Geometry check sheet. Reference: the model listing, model coordinates, mm. Face numbers are marked on the shaded views. A direction names the side the tool comes from. Coordinates: 2 decimals unless noted, no trailing zeros. Order: outer loops, then holes, each group sorted by start corner. A loop starts at its lowest first (then second) coordinate and runs counter-clockwise, first axis right, second up. Notation, with made-up numbers: (19, 74) - (64, 74) arc R24 cw to (64, 97) - close; hole circle Ø9 at (15, -25.75). An arc over 180 degrees is marked (long way). Put each result on its own line as item: value.
from build123d import *

# Parameters (mm, degrees)
SKETCH4_R           = 37.5
BOSS_EXTRUDE2_DEPTH = 5
SKETCH5_R           = 8.5
CUT_EXTRUDE1_DEPTH  = 54.268189382
BOSS_EXTRUDE3_DEPTH = 4.7
SKETCH1_R           = 37.5
SKETCH1_R_2         = 26.5
CUT_EXTRUDE2_DEPTH  = 57.626164447


with BuildPart() as part:
    # Sketch4 → Boss-Extrude2 (new body)
    with BuildSketch(Plane.XY):
        Circle(SKETCH4_R)
    extrude(amount=BOSS_EXTRUDE2_DEPTH)

    # Sketch5 → Cut-Extrude1 (cut, through all)
    with BuildSketch(Plane.XY.offset(5)):
        Circle(SKETCH5_R)
    extrude(amount=-CUT_EXTRUDE1_DEPTH, mode=Mode.SUBTRACT)

    # Sketch6 → Boss-Extrude3 (add, symmetric)
    with BuildSketch(Plane(origin=(0, 0, 0), x_dir=(1, 0, 0), z_dir=(0, 1, 0))):
        Polygon((26.5, 0), (20.712132034, 0), (23.65, 2.937867966), (23.65, 14.562132034), (21.65, 16.562132034), (21.65, 19.85), (26.5, 19.85), align=None)
    boss_extrude3 = extrude(amount=BOSS_EXTRUDE3_DEPTH, both=True)

    # Mirror1: Boss-Extrude3 across plane
    add(boss_extrude3.mirror(Plane(origin=(0, 0, 0), x_dir=(0, 0, 1), z_dir=(1, 0, 0))))

    # Sketch1 → Cut-Extrude2 (cut, through all)
    with BuildSketch(Plane.XY):
        Circle(SKETCH1_R)
        Circle(SKETCH1_R_2, mode=Mode.SUBTRACT)
    extrude(amount=-CUT_EXTRUDE2_DEPTH, mode=Mode.SUBTRACT)


solid = part.part
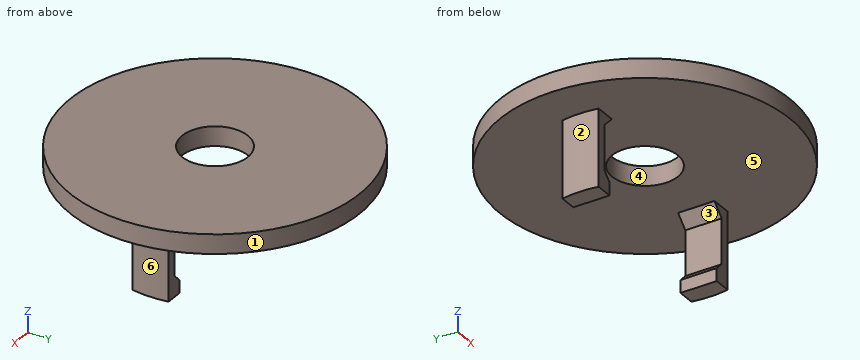
Q1. Thickness scan on L1, parallel to Y at x = 0, z = 3.85; L2, parallel to Z at x = 32, y = 1; L3, parallel to X at y = -1, z = -16.5. Record the ranges inside material, lowest first. Write a range as [from, to].
Answer block:
L1: y = [-37.5, -8.5], [8.5, 37.5]
L2: z = [0, 5]
L3: x = [-26.48, -21.71], [21.71, 26.48]
Q2. Section check B-B on z = -9.75. Record the boundary of the cut face in (x, y).
Answer block:
outline: (-26.08, -4.7) - (-23.65, -4.7) - (-23.65, 4.7) - (-26.08, 4.7) arc R26.5 ccw to start; (23.65, -4.7) - (26.08, -4.7) arc R26.5 ccw to (26.08, 4.7) - (23.65, 4.7) - close
Q3. Draft check along Y on the marked faces 4, 5 and 6. Enter one of: pulls with the +Y half, pulls with the -Y half, needs draft (parallel to the pull), parting line crosses it, or undercut.
Answer block:
face 4: undercut
face 5: needs draft
face 6: parting line crosses it
Q4. Section check A-A on x = 0. Record the boundary of the cut face in (y, z), then the cut area to 3 significant figures.
Answer block:
outline: (-37.5, 0) - (-8.5, 0) - (-8.5, 5) - (-37.5, 5) - close; (8.5, 0) - (37.5, 0) - (37.5, 5) - (8.5, 5) - close
area: 290 mm^2
Q5. Depth check by flat-ended pin: pin 1 Ø2.5 at (x, z) = (22.5, -7.5) entering from +Y; pin 2 Ø1.6 at (x, z) = (-24.5, -9.5) entering from -Y; pin 3 Ø12 at (x, y) = (-21.5, -27) entering from -Z; pin 4 Ø5 at (y, z) = (-19.5, -4.5) entering from -X. Enter the tip coordinate at first touch or a pass-through.
Answer block:
pin 1: stops at y = 4.7
pin 2: stops at y = -4.7
pin 3: stops at z = 0
pin 4: passes through
Q6. Section check C-C on y = 0. Record the boundary of the cut face in (x, z), then the cut area to 3 significant figures.
Answer block:
outline: (-37.5, 0) - (-26.5, 0) - (-26.5, -19.85) - (-21.65, -19.85) - (-21.65, -16.56) - (-23.65, -14.56) - (-23.65, -2.94) - (-20.71, 0) - (-8.5, 0) - (-8.5, 5) - (-37.5, 5) - close; (8.5, 0) - (20.71, 0) - (23.65, -2.94) - (23.65, -14.56) - (21.65, -16.56) - (21.65, -19.85) - (26.5, -19.85) - (26.5, 0) - (37.5, 0) - (37.5, 5) - (8.5, 5) - close
area: 429 mm^2
Q7. Access from +Z, -Z, +X, -X, +Y, -Y to the whole of each face (thin tool, end or side, straight path). Record for the marked faces 1, 2 and 3.
Answer block:
face 1: +Z, -Z
face 2: -Z, -X
face 3: +Y, -Y
Q8. Section check D-D on y = 30. Record the boundary of the cut face in (x, z), then the cut area to 3 significant figures.
Answer block:
outline: (-22.5, 0) - (22.5, 0) - (22.5, 5) - (-22.5, 5) - close
area: 225 mm^2
